Here's how the part is built. I have some questions about the finished solid (model axes, mm). A direction names the side the tool comes from. Round coordinates to 2 decimals unless told otherwise and drop trailing zeros. Loops run counter-clockwise (first coordinate to the right, second up) from the corner with the lowest first, then second, coordinate; pieces in that order, holes last. Notation, with made-up numbers: M 12,7 L 18,7 A28 ccw 18,31 Z; hole C 59,27.5 d6. An arc over 180 degrees is marked long. Answer as a JSON object with one key per item and string values.
from build123d import *

# Parameters (mm, degrees)
SKETCH_1_R          = 1.5
SKETCH_1_R_2        = 1.6
EXTRUDE_1_DEPTH     = 1.5
CHAMFER_1_SIZE      = 1.5
SKETCH_2_R          = 0.75
CUT_EXTRUDE_1_DEPTH = 28.684874976
CUT_EXTRUDE_2_DEPTH = 28.684874976
FILLET_1_R          = 2.5
FILLET_2_R          = 1


with BuildPart() as part:
    # 草图1 → 凸台-拉伸1 (new, symmetric)
    with BuildSketch(Plane.XY):
        with BuildLine():
            Line((-7.5, -12), (-3.5, -12))
            Line((-3.5, -12), (-3.5, 0))
            ThreePointArc((-3.5, 0), (-1.997674375, 2.873899283), (1.219598337, 3.280637117))
            Line((1.219598337, 3.280637117), (12.609663209, -0.953694105))
            ThreePointArc((12.609663209, -0.953694105), (14.628222296, -3.204119106), (13.92040375, -6.143164253))
            Line((13.92040375, -6.143164253), (-0.114583662, -22.143164253))
            ThreePointArc((-0.114583662, -22.143164253), (-3.157233879, -23.194243112), (-5.61180939, -21.111565466))
            Line((-5.61180939, -21.111565466), (-8.439692621, -13.342020143))
            ThreePointArc((-8.439692621, -13.342020143), (-8.319152044, -12.426423564), (-7.5, -12))
        make_face()
        Circle(SKETCH_1_R, mode=Mode.SUBTRACT)
        with Locations((-2.557808372, -20)):
            Circle(SKETCH_1_R_2, mode=Mode.SUBTRACT)
        with Locations((11.477179039, -4)):
            Circle(SKETCH_1_R_2, mode=Mode.SUBTRACT)
    extrude(amount=EXTRUDE_1_DEPTH, both=True)

    # 倒角1
    chamfer_1_edges = [part.edges().sort_by_distance(p)[0] for p in [
        (-4.157808372, -20, 1.5),
    ]]
    chamfer(chamfer_1_edges, length=CHAMFER_1_SIZE)

    # 草图2 → 切除-拉伸1 (cut, through all)
    with BuildSketch(Plane.XY.offset(1.5)):
        with Locations((-4.25, -12)):
            Circle(SKETCH_2_R)
    extrude(amount=-CUT_EXTRUDE_1_DEPTH, mode=Mode.SUBTRACT)

    # 草图3 → 切除-拉伸2 (cut, through all)
    with BuildSketch(Plane.XY.offset(1.5)):
        with BuildLine():
            Line((5.807426852, -7.5), (12.73020546, -7.5))
            Line((12.73020546, -7.5), (-0.114583662, -22.143164253))
            ThreePointArc((-0.114583662, -22.143164253), (0.219636548, -21.687690646), (0.469932731, -21.181221322))
            Line((0.469932731, -21.181221322), (5.807426852, -7.5))
        make_face()
    extrude(amount=-CUT_EXTRUDE_2_DEPTH, mode=Mode.SUBTRACT)

    # 圆角1
    fillet_1_edges = [part.edges().sort_by_distance(p)[0] for p in [
        (5.807426852, -7.5, 0),
    ]]
    fillet(fillet_1_edges, radius=FILLET_1_R)

    # 圆角2
    fillet_2_edges = [part.edges().sort_by_distance(p)[0] for p in [
        (12.73020546, -7.5, 0),
    ]]
    fillet(fillet_2_edges, radius=FILLET_2_R)


solid = part.part
Item 1: For faces 5 (the face through (-6, -12, 0)), 6 (the face through (10, -7.5, 0)), 7 (the face through (-4.27, -12.75, 0.02)), which set-ups out of +Z, -Z, +X, -X, +Y, -Y let a thin tool reach every point of the face, with its end or its side?
Solution:
{"face 5": "+Z, -Z, -X, +Y", "face 6": "+Z, -Z, +X, -Y", "face 7": "+Z, -Z, +Y"}
Item 2: If I drill on L1, parallel to Y at x = -1.25, z = -0.2; L2, parallel to Y at x = -0.5, z = -1.25; L3, parallel to Y at x = -3, z = 0.3, over which ranges is the centre line in solid material (lowest first)? Write a range as from..to.
Solution:
{"L1": "y = -22.98..-20.92, -19.08..-0.83, 0.83..3.27", "L2": "y = -22.52..-1.41, 1.41..3.46", "L3": "y = -23.22..-21.85, -18.15..1.8"}
Item 3: I want a section at A-A on y = -4. List the corners of the cut face in (x, z) for me.
Solution:
{"outline": "M -3.5,-1.5 L 9.88,-1.5 L 9.88,1.5 L -3.5,1.5 Z; M 13.08,-1.5 L 14.73,-1.5 L 14.73,1.5 L 13.08,1.5 Z"}
Item 4: For P1, Ø0.9, axis at x = 10.5, z = 0.5, coming from the -Y side; P2, Ø0.8, axis at x = -6.5, z = -0.5, coming from the +Y side; P3, Ø2.5, axis at x = 11.48, y = -4, coming from the -Z side, each with a flat end and sliding along its axis, tell me the tip position at first contact or that it passes through.
Solution:
{"P1": "stops at y = -7.5", "P2": "stops at y = -12", "P3": "passes through"}
Item 5: I want a section at C-C on y = -10.5. List the corners of the cut face in (x, z) for me, plus the area to 3 significant figures.
Solution:
{"outline": "M -3.5,-1.5 L 4.64,-1.5 L 4.64,1.5 L -3.5,1.5 Z", "area": "24.4 mm2"}
Item 6: We'd pull the mould along Y, two halves only. Please class faces 1 (the face through (13.481, -6.644, 0.021)), 2 (the face through (-2.766, -18.414, -0.76)), 3 (the face through (-2.036, 2.847, 0.021)), 4 (the face through (9.88, -3.93, -0.02)): +Y half, -Y half, draft (parallel to the pull), parting line (faces both ways), or undercut.
Solution:
{"face 1": "-Y half", "face 2": "undercut", "face 3": "+Y half", "face 4": "undercut"}
Item 7: I want a section at B-B on x = 9. List the corners of the cut face in (y, z) for me, plus the area to 3 significant figures.
Solution:
{"outline": "M -7.5,-1.5 L 0.39,-1.5 L 0.39,1.5 L -7.5,1.5 Z", "area": "23.7 mm2"}
